Here's how the part is built. I have some questions about the finished solid (model axes, mm). Face numbers are marked on the shaded views. A direction names the side the tool comes from. Give positions to 0.01 mm unless a question says otherwise; leave off trailing zeros. Write each loop counter-clockwise with the first axis right and the second up, starting at its lowest first coordinate (ties: lowest second). Pieces come first, ordered by that corner, then holes. Notation, with made-up numbers: (16.25, -38) -> (48.25, -38) arc R34 ccw to (48.25, -1) -> close; hole circle Ø6 at (81.5, 28.25). An arc over 180 degrees is marked (long way). Put each result on its own line as item: value. Start each with the question number.
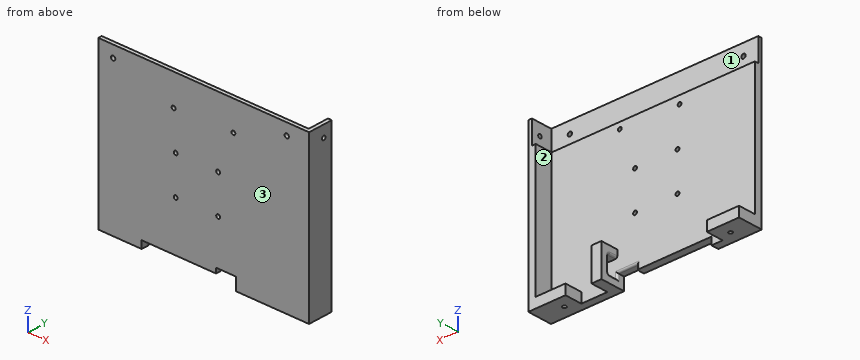
from build123d import *

# Parameters (mm, degrees)
BOSS_EXTRUDE1_DEPTH = 6
SKETCH2_W           = 26
SKETCH2_H           = 8
SKETCH2_W_2         = 30
BOSS_EXTRUDE2_DEPTH = 14
SKETCH3_R           = 1.55
CUT_EXTRUDE1_DEPTH  = 9
SKETCH4_W           = 170
SKETCH4_H           = 18.5
CUT_EXTRUDE2_DEPTH  = 3
SKETCH5_R           = 1.75
CUT_EXTRUDE3_DEPTH  = 3
BOSS_EXTRUDE3_REACH = 22
SKETCH8_R           = 1.55
CUT_EXTRUDE4_DEPTH  = 4
CUT_EXTRUDE5_REACH  = 8
SKETCH9_W           = 16
SKETCH9_H           = 10
SKETCH10_W          = 8
SKETCH10_H          = 26
BOSS_EXTRUDE4_DEPTH = 14
CUT_EXTRUDE6_REACH  = 121
FILLET1_R           = 1.5
SKETCH12_R          = 1.55
CUT_EXTRUDE7_DEPTH  = 14
CUT_EXTRUDE8_REACH  = 8
SKETCH13_R          = 1.55


with BuildPart() as part:
    # Sketch1 → Boss-Extrude1 (new body)
    with BuildSketch(Plane(origin=(0, 0, 0), x_dir=(1, 0, 0), z_dir=(0, 1, 0))):
        Polygon((-85, 65.375), (-85, -65.375), (85, -65.375), (85, 65.375), (10, 65.375), (10, 59.375), (-50, 59.375), (-50, 65.375), align=None)
    extrude(amount=BOSS_EXTRUDE1_DEPTH)

    # Sketch2 → Boss-Extrude2 (add)
    with BuildSketch(Plane(origin=(0, 6, 0), x_dir=(1, 0, 0), z_dir=(0, 1, 0))):
        with Locations((-72, 61.375)):
            Rectangle(SKETCH2_W, SKETCH2_H)
        with Locations((70, 61.375)):
            Rectangle(SKETCH2_W_2, SKETCH2_H)
    extrude(amount=BOSS_EXTRUDE2_DEPTH)

    # Sketch3 → Cut-Extrude1 (cut, through all)
    with BuildSketch(Plane.XY.offset(-57.375)):
        with Locations((-69, 10)):
            Circle(SKETCH3_R)
        with Locations((65, 10)):
            Circle(SKETCH3_R)
    extrude(amount=-CUT_EXTRUDE1_DEPTH, mode=Mode.SUBTRACT)

    # Sketch4 → Cut-Extrude2 (cut)
    with BuildSketch(Plane(origin=(0, 6, 0), x_dir=(1, 0, 0), z_dir=(0, 1, 0))):
        with Locations((0, -56.125)):
            Rectangle(SKETCH4_W, SKETCH4_H)
    extrude(amount=-CUT_EXTRUDE2_DEPTH, mode=Mode.SUBTRACT)

    # Sketch5 → Cut-Extrude3 (cut)
    with BuildSketch(Plane(origin=(0, 3, 0), x_dir=(1, 0, 0), z_dir=(0, 1, 0))):
        with Locations((-73, -56.125)):
            Circle(SKETCH5_R)
        with Locations((67, -56.125)):
            Circle(SKETCH5_R)
    extrude(amount=-CUT_EXTRUDE3_DEPTH, mode=Mode.SUBTRACT)

    # Sketch7 → Boss-Extrude3 (add, up to next)
    with BuildSketch(Plane(origin=(0, 20, 0), x_dir=(1, 0, 0), z_dir=(0, 1, 0)), mode=Mode.PRIVATE) as boss_extrude3_sk1:
        Polygon((85, -65.375), (85, 57.375), (79, 57.375), (79, -46.875), (82, -46.875), (82, -65.375), align=None)
    boss_extrude3_tool1 = extrude(boss_extrude3_sk1.sketch, amount=-BOSS_EXTRUDE3_REACH, mode=Mode.PRIVATE) - part.part
    add(boss_extrude3_tool1.solids().sort_by_distance((82.122247, 20, -0.248073))[0])

    # Sketch8 → Cut-Extrude4 (cut, through all)
    with BuildSketch(Plane.ZY.offset(-82)):
        with Locations((56.125, 13)):
            Circle(SKETCH8_R)
    extrude(amount=-CUT_EXTRUDE4_DEPTH, mode=Mode.SUBTRACT)

    # Sketch9 → Cut-Extrude5 (cut, up to next)
    with BuildSketch(Plane(origin=(0, 6, 0), x_dir=(1, 0, 0), z_dir=(0, 1, 0)), mode=Mode.PRIVATE) as cut_extrude5_sk1:
        with Locations((18, 60.375)):
            Rectangle(SKETCH9_W, SKETCH9_H)
    cut_extrude5_tool1 = extrude(cut_extrude5_sk1.sketch, amount=-CUT_EXTRUDE5_REACH, mode=Mode.PRIVATE) & part.part
    add(cut_extrude5_tool1.solids().sort_by_distance((18, 6, -60.375))[0], mode=Mode.SUBTRACT)

    # Sketch10 → Boss-Extrude4 (add)
    with BuildSketch(Plane(origin=(0, 6, 0), x_dir=(1, 0, 0), z_dir=(0, 1, 0))):
        with Locations((30, 52.375)):
            Rectangle(SKETCH10_W, SKETCH10_H)
    extrude(amount=BOSS_EXTRUDE4_DEPTH)

    # Sketch11 → Cut-Extrude6 (cut, up to next)
    with BuildSketch(Plane(origin=(34, 0, 0), x_dir=(0, 0, -1), z_dir=(1, 0, 0)), mode=Mode.PRIVATE) as cut_extrude6_sk1:
        Polygon((45.375, 12), (45.375, 6), (59.375, 6), (59.375, 12), (59.375, 14), (45.375, 14), align=None)
    cut_extrude6_tool1 = extrude(cut_extrude6_sk1.sketch, amount=-CUT_EXTRUDE6_REACH, mode=Mode.PRIVATE) & part.part
    add(cut_extrude6_tool1.solids().sort_by_distance((34, 10, -52.375))[0], mode=Mode.SUBTRACT)

    # Fillet1
    fillet1_edges = [part.edges().sort_by_distance(p)[0] for p in [
        (26, 6, -57.375),
        (18, 6, -55.375),
        (10, 6, -57.375),
        (26, 10, -45.375),
        (26, 14, -52.375),
        (26, 10, -59.375),
        (34, 10, -59.375),
        (34, 14, -52.375),
        (34, 10, -45.375),
        (30, 14, -45.375),
        (30, 14, -59.375),
    ]]
    fillet(fillet1_edges, radius=FILLET1_R)

    # Sketch12 → Cut-Extrude7 (cut)
    with BuildSketch(Plane(origin=(0, 6, 0), x_dir=(1, 0, 0), z_dir=(0, 1, 0))):
        with Locations((24, -41.875)):
            Circle(SKETCH12_R)
        with Locations((-24.26, -40.575)):
            Circle(SKETCH12_R)
    extrude(amount=-CUT_EXTRUDE7_DEPTH, mode=Mode.SUBTRACT)

    # Sketch13 → Cut-Extrude8 (cut, up to next)
    with BuildSketch(Plane(origin=(0, 6, 0), x_dir=(1, 0, 0), z_dir=(0, 1, 0)), mode=Mode.PRIVATE) as cut_extrude8_sk1:
        with Locations((11.685222517, 19.828524859)):
            Circle(SKETCH13_R)
    cut_extrude8_tool1 = extrude(cut_extrude8_sk1.sketch, amount=-CUT_EXTRUDE8_REACH, mode=Mode.PRIVATE) & part.part
    add(cut_extrude8_tool1.solids().sort_by_distance((11.685223, 6, -19.828525))[0], mode=Mode.SUBTRACT)
    # Sketch13 → Cut-Extrude8 (cut, up to next)
    with BuildSketch(Plane(origin=(0, 6, 0), x_dir=(1, 0, 0), z_dir=(0, 1, 0)), mode=Mode.PRIVATE) as cut_extrude8_sk2:
        with Locations((-22.560396417, 19.828524859)):
            Circle(SKETCH13_R)
    cut_extrude8_tool2 = extrude(cut_extrude8_sk2.sketch, amount=-CUT_EXTRUDE8_REACH, mode=Mode.PRIVATE) & part.part
    add(cut_extrude8_tool2.solids().sort_by_distance((-22.560396, 6, -19.828525))[0], mode=Mode.SUBTRACT)
    # Sketch13 → Cut-Extrude8 (cut, up to next)
    with BuildSketch(Plane(origin=(0, 6, 0), x_dir=(1, 0, 0), z_dir=(0, 1, 0)), mode=Mode.PRIVATE) as cut_extrude8_sk3:
        with Locations((11.685222517, -10.544533108)):
            Circle(SKETCH13_R)
    cut_extrude8_tool3 = extrude(cut_extrude8_sk3.sketch, amount=-CUT_EXTRUDE8_REACH, mode=Mode.PRIVATE) & part.part
    add(cut_extrude8_tool3.solids().sort_by_distance((11.685223, 6, 10.544533))[0], mode=Mode.SUBTRACT)
    # Sketch13 → Cut-Extrude8 (cut, up to next)
    with BuildSketch(Plane(origin=(0, 6, 0), x_dir=(1, 0, 0), z_dir=(0, 1, 0)), mode=Mode.PRIVATE) as cut_extrude8_sk4:
        with Locations((-22.560396417, -10.544533108)):
            Circle(SKETCH13_R)
    cut_extrude8_tool4 = extrude(cut_extrude8_sk4.sketch, amount=-CUT_EXTRUDE8_REACH, mode=Mode.PRIVATE) & part.part
    add(cut_extrude8_tool4.solids().sort_by_distance((-22.560396, 6, 10.544533))[0], mode=Mode.SUBTRACT)


solid = part.part
1) I want a section at C-C, the plane z = 52.5. Write out the boundary of the cut face in (x, y).
2) I need wall thicknesses on probe 1 along X at (y, z) = (15.25, -57); probe 2 along Z at (x, y) = (-24.26, 1.4) (3 decimals); probe 3 along Z at (x, y) = (-37, 1.5) (3 decimals). Which ranges of each line are inside material? Lowest first, please.
3) I want a section at B-B, the plane x = 38. Write out the boundary of the cut face in (y, z) (3 decimals), and give its area (3 significant figures).
4) Which directions (+Z, -Z, +X, -X, +Y, -Y) give clear straight access to the entire face, cutting with the end or side of a thin tool? Please do the marked faces 1, 2 and 3.
5) I want a section at D-D, the plane x = 16.5. Write out the boundary of the cut face in (y, z) (3 decimals), and give its area (3 significant figures).
6) I want a section at A-A, the plane x = -73. Write out the boundary of the cut face in (y, z) (3 decimals), and give its area (4 significant figures).
7) I'm going to push flat-ended pins straight in: pin 1 Ø2 at (x, y) = (-26.5, 8.5) entering from -Z; pin 2 Ø8 at (y, z) = (17, -42) entering from -X; pin 3 Ø12 at (x, z) = (-48.5, 12) entering from +Y; pin 4 Ø6.5 at (x, y) = (29.5, 10.5) entering from +Z (3 decimals). Where does each tip first touch, or does it pass through?
Established:
1. outline: (-85, 0) -> (85, 0) -> (85, 20) -> (82, 20) -> (82, 3) -> (-85, 3) -> close
2. probe 1: x = 26.02 to 33.98, 79 to 85
2. probe 2: z = -59.375 to 39.025, 42.125 to 65.375
2. probe 3: z = -59.375 to 65.375
3. outline: (0, -65.375) -> (6, -65.375) -> (6, 46.875) -> (3, 46.875) -> (3, 65.375) -> (0, 65.375) -> close
3. area: 729 mm2
4. face 1: +Z, -X, +Y
4. face 2: +Z, +Y
4. face 3: +Z, -Z, +X, -X, -Y
5. outline: (0, -55.375) -> (4.5, -55.375) arc R1.5 ccw to (6, -53.875) -> (6, 46.875) -> (3, 46.875) -> (3, 65.375) -> (0, 65.375) -> close
5. area: 669 mm2
6. outline: (0, -65.375) -> (20, -65.375) -> (20, -57.375) -> (6, -57.375) -> (6, 46.875) -> (3, 46.875) -> (3, 54.375) -> (0, 54.375) -> close; (0, 57.875) -> (3, 57.875) -> (3, 65.375) -> (0, 65.375) -> close
6. area: 830.5 mm2
7. pin 1: passes through
7. pin 2: stops at x = 26
7. pin 3: stops at y = 6
7. pin 4: stops at z = -39.375
